Job drawing, mm, ordinate dimensions from the low corner. One solid piece. Give positions to 0.01 mm unless a question says otherwise; leave off trailing zeros. Write each loop counter-clockwise with the first axis right and the second up, starting at its lowest first coordinate (ties: lowest second). Pieces come first, ordered by that corner, then holes. Notation, with made-up numbers: (0.25, 13) -> (27.25, 13) arc R12 cw to (27.25, 36) -> close; hole circle Ø1 at (-25.5, 46). An arc over 180 degrees is marked (long way). Put each result on its own line as item: value. Start each with the question number.
Item 1: Flat gauge pin, fed straight in: pin 1 Ø10 at (y, z) = (65.5, 20) entering from -X. Where does the tip first touch, or does it go through?
Item 2: Drill centre lines: line 1 along X through (y, z) = (66, 27.5); line 2 along Y through (x, z) = (39, 28); line 3 along X through (y, z) = (52, 29). Where is each one in solid material? Low to high.
Item 3: Slice it at A-A, the plane x = 65. List the corners of the cut face in (y, z), plus the area to 3 significant figures.
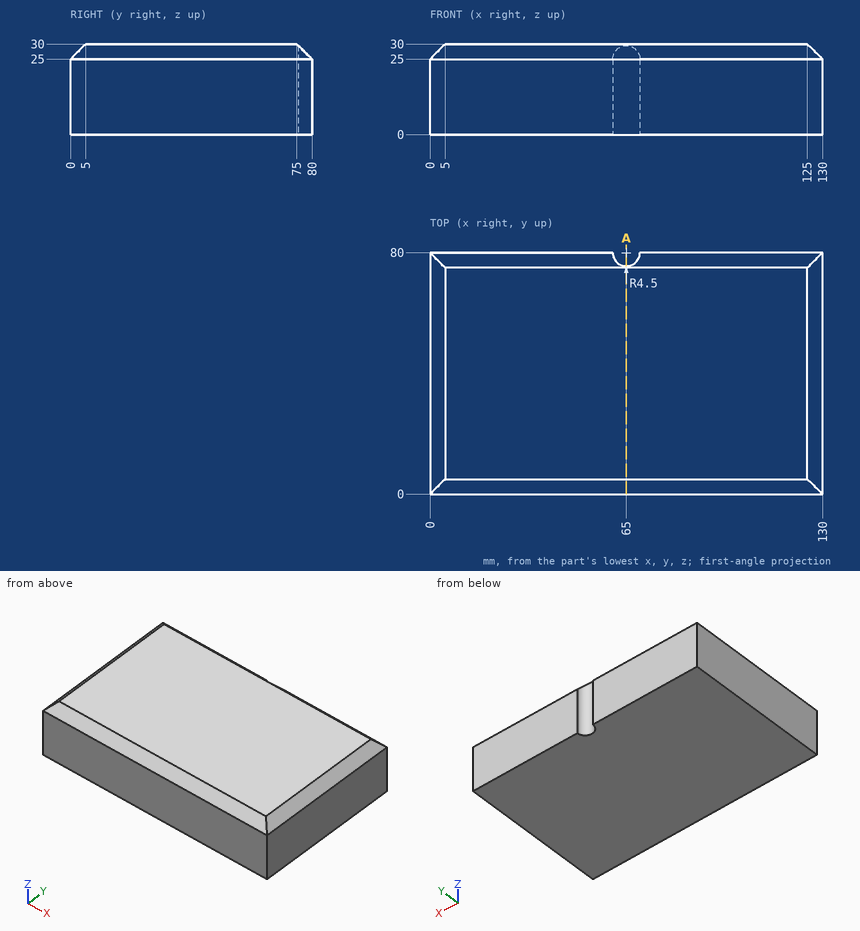
Values follow:
1. pin 1: x = 0
2. line 1: 2.5 to 127.5
2. line 2: 3 to 77
2. line 3: 4 to 126
3. outline: (0, 0) -> (75.5, 0) -> (75.5, 29.5) -> (75, 30) -> (5, 30) -> (0, 25) -> close
3. area: 2,250 mm2
